Part model, mm, in its own coordinate system. Face numbers are marked on the shaded views. A direction names the side the tool comes from. Round coordinates to 2 decimals unless told otherwise and drop trailing zeros. Loops run counter-clockwise (first coordinate to the right, second up) from the corner with the lowest first, then second, coordinate; pieces in that order, holes last.
from build123d import *

# Parameters (mm, degrees)
EXTRUDE_1_DEPTH = 100
EXTRUDE_2_DEPTH = 20


with BuildPart() as part:
    # 草图1 → 凸台-拉伸1 (new, symmetric)
    with BuildSketch(Plane.XY):
        with BuildLine():
            Line((-10, 15), (10, 15))
            ThreePointArc((10, 15), (25, 0), (10, -15))
            Line((10, -15), (-10, -15))
            ThreePointArc((-10, -15), (-25, 0), (-10, 15))
        make_face()
    extrude(amount=EXTRUDE_1_DEPTH, both=True)

    # 草图2 → 凸台-拉伸2 (add)
    with BuildSketch(Plane(origin=(0, 0, -100), x_dir=(-1, 0, 0), z_dir=(0, 0, -1))):
        with BuildLine():
            Line((-5, 5), (5, 5))
            ThreePointArc((5, 5), (10, 0), (5, -5))
            Line((5, -5), (-5, -5))
            ThreePointArc((-5, -5), (-10, 0), (-5, 5))
        make_face()
    extrude(amount=EXTRUDE_2_DEPTH)


solid = part.part
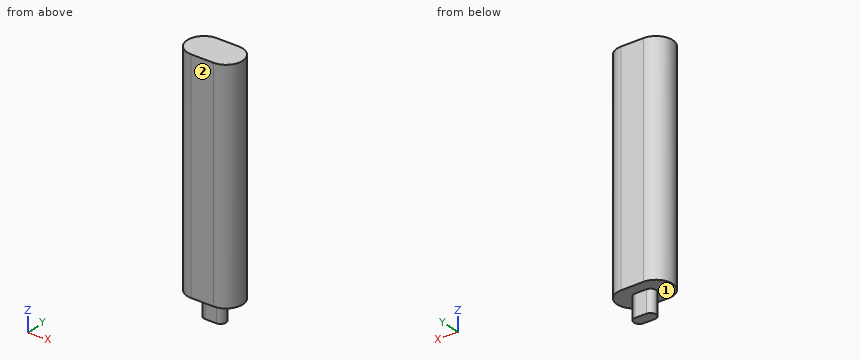
1) Drop flat-ended pins along their axis: pin 1 Ø8 at (y, z) = (7.5, 10.5) entering from +X; pin 2 Ø5 at (x, z) = (19.5, 63) entering from -Y; pin 3 Ø8 at (x, z) = (2, -113) entering from -Y. Give the stop position or say it passes through.
Values:
pin 1: stops at x = 24.59
pin 2: stops at y = -13.27
pin 3: stops at y = -5
2) Tool access for the marked faces 1 and 2: list every direction of +Z, -Z, +X, -X, +Y, -Y with a clear straight run to the whole face (end or side of a thin tool).
Values:
face 1: -Z
face 2: +Z, -Z, +X, -X, -Y
3) Wall check: line 1 along Y through (x, z) = (-11, -32); line 2 along Z through (x, y) = (4.5, 14.5); line 3 along X through (y, z) = (-0.5, 15.5). Give the ranges that are in metal, low to high.
Values:
line 1: y = -14.97 to 14.97
line 2: z = -100 to 100
line 3: x = -24.99 to 24.99
4) Slice it at A-A, the plane y = 0. Give the cut face in (x, z), then the cut area to 3 significant figures.
Values:
outline: (-25, -100) - (-10, -100) - (-10, -120) - (10, -120) - (10, -100) - (25, -100) - (25, 100) - (-25, 100) - close
area: 10,400 mm2
5) Slice it at C-C, the plane y = -12. Give the cut face in (x, z), then the cut area to 3 significant figures.
Values:
outline: (-19, -100) - (19, -100) - (19, 100) - (-19, 100) - close
area: 7,600 mm2
6) Slice it at B-B, the plane z = -89.5. Give the cut face in (x, y), then the cut area to 3 significant figures.
Values:
outline: (-10, -15) - (10, -15) arc R15 ccw to (10, 15) - (-10, 15) arc R15 ccw to start
area: 1,310 mm2
